from build123d import *

# Parameters (mm, degrees)
SKETCH1_W                    = 165
SKETCH1_H                    = 60
BOSS_EXTRUDE1_DEPTH          = 18
SKETCH3_R                    = 20
CUT_EXTRUDE2_DEPTH           = 18
F_4_0_4_DIAMETER_HOLE1_D     = 4
F_4_0_4_DIAMETER_HOLE1_DEPTH = 30
F_4_0_4_DIAMETER_HOLE1_TIP   = 1.201721238
F_6_0_6_DIAMETER_HOLE2_D     = 6
F_6_0_6_DIAMETER_HOLE2_DEPTH = 14
F_5_0_5_DIAMETER_HOLE1_D     = 5


with BuildPart() as part:
    # Sketch1 → Boss-Extrude1 (new body)
    with BuildSketch(Plane.XY):
        Rectangle(SKETCH1_W, SKETCH1_H)
    extrude(amount=BOSS_EXTRUDE1_DEPTH)

    # Sketch3 → Cut-Extrude2 (cut)
    with BuildSketch(Plane.XY.offset(18)):
        with Locations((0, -5)):
            Circle(SKETCH3_R)
    extrude(amount=-CUT_EXTRUDE2_DEPTH, mode=Mode.SUBTRACT)

    # Ø4.0 (4) Diameter Hole1
    with Locations(Plane(origin=(0, -30, 0), x_dir=(-1, 0, 0), z_dir=(0, -1, 0))):
        with Locations((57.5, -9), (-57.5, -9)):
            Hole(F_4_0_4_DIAMETER_HOLE1_D / 2, depth=F_4_0_4_DIAMETER_HOLE1_DEPTH)
            with Locations((0, 0, -(F_4_0_4_DIAMETER_HOLE1_DEPTH + F_4_0_4_DIAMETER_HOLE1_TIP / 2))):  # 118° drill point
                Cone(0, F_4_0_4_DIAMETER_HOLE1_D / 2, F_4_0_4_DIAMETER_HOLE1_TIP, mode=Mode.SUBTRACT)

    # Ø6.0 (6) Diameter Hole2
    with Locations(Plane.XY.offset(18)):
        with Locations((73.5, 10), (-73.5, 10)):
            Hole(F_6_0_6_DIAMETER_HOLE2_D / 2, depth=F_6_0_6_DIAMETER_HOLE2_DEPTH)

    # Ø5.0 (5) Diameter Hole1 (through all)
    with Locations(Plane(origin=(0, 0, 0), x_dir=(-1, 0, 0), z_dir=(0, 0, -1))):
        with Locations((-46.05, 9.95), (-46.05, -22.05), (45.95, 9.95), (45.95, -22.05)):
            Hole(F_5_0_5_DIAMETER_HOLE1_D / 2)


solid = part.part
Check sheet for the modelled part. Datum: model origin and axes. Units: mm. A direction names the side the tool comes from. Round coordinates to 2 decimals unless told otherwise and drop trailing zeros. Loops run counter-clockwise (first coordinate to the right, second up) from the corner with the lowest first, then second, coordinate; pieces in that order, holes last.
1. Sectioned sample at D-D on z = 13. Record the boundary of the cut face in (x, y), and give its area (3 significant figures).
2. Gauge pin test, flat ends, axial feed: pin 1 Ø12 at (x, y) = (6, -16) entering from -Z; pin 2 Ø3.5 at (x, z) = (-57.5, 9) entering from -Y; pin 3 Ø3 at (x, y) = (-74, 11) entering from +Z. Record the tip position at first contact, or that the pin passes through.
3. Sectioned sample at B-B on x = -45.95. Record the boundary of the cut face in (y, z).
4. Mould release check, pull along X, two halves, no side actions. Record for faces 1 (the flat face through (82.5, 0, 9)), 2 (the flat face through (-82.5, 0, 9)), 3 (the flat face through (-19.5, 0.4, 0)), 4 (the conical face through (57.169, 0.993, 8.896)): released by +X, released by -X, zero draft, split by the parting line, or undercut.
5. Scan lines: probe 1 along Y at (x, z) = (-45.95, 6.25); probe 2 along Z at (x, y) = (-57.5, -12); probe 3 along Y at (x, z) = (0, 6.5). Record each from-to range of solid material in increasing order.
6. Set-up check for faces 5 (the cylindrical face through (-55.592, -14.79, 8.399)), 6 (the flat face through (-1, 30, 9)), 7 (the cylindrical face through (75.9, 8.2, 10.9)): record each of +Z, -Z, +X, -X, +Y, -Y from which the full face is reachable in a straight line by a thin tool's end or side.
7. Sectioned sample at A-A on y = -5. Record the boundary of the cut face in (x, z).
8. Sectioned sample at C-C on z = 2.5. Record the boundary of the cut face in (x, y).
Recorded:
1. outline: (-82.5, -30) - (82.5, -30) - (82.5, 30) - (-82.5, 30) - close; hole circle Ø6 at (-73.5, 10); hole circle Ø5 at (-45.95, -22.05); hole circle Ø5 at (-45.95, 9.95); hole circle Ø40 at (0, -5); hole circle Ø5 at (46.05, -22.05); hole circle Ø5 at (46.05, 9.95); hole circle Ø6 at (73.5, 10)
1. area: 8,510 mm2
2. pin 1: passes through
2. pin 2: stops at y = 0.15
2. pin 3: stops at z = 4
3. outline: (-30, 0) - (-24.55, 0) - (-24.55, 18) - (-30, 18) - close; (-19.55, 0) - (7.45, 0) - (7.45, 18) - (-19.55, 18) - close; (12.45, 0) - (30, 0) - (30, 18) - (12.45, 18) - close
4. face 1: released by +X
4. face 2: released by -X
4. face 3: zero draft
4. face 4: undercut
5. probe 1: y = -30 to -24.55, -19.55 to 7.45, 12.45 to 30
5. probe 2: z = 0 to 7, 11 to 18
5. probe 3: y = -30 to -25, 15 to 30
6. face 5: -Y
6. face 6: +Z, -Z, +X, -X, +Y
6. face 7: +Z
7. outline: (-82.5, 0) - (-20, 0) - (-20, 18) - (-82.5, 18) - close; (20, 0) - (82.5, 0) - (82.5, 18) - (20, 18) - close; hole circle Ø4 at (-57.5, 9); hole circle Ø4 at (57.5, 9)
8. outline: (-82.5, -30) - (82.5, -30) - (82.5, 30) - (-82.5, 30) - close; hole circle Ø5 at (-45.95, -22.05); hole circle Ø5 at (-45.95, 9.95); hole circle Ø40 at (0, -5); hole circle Ø5 at (46.05, -22.05); hole circle Ø5 at (46.05, 9.95)
